For this review, use the dimensioned drawing (mm, ordinates from the lowest corner) and the shaded views. Give positions to 0.01 mm unless a question says otherwise; leave off trailing zeros. Order: outer loops, then holes, each group sorted by start corner. A loop starts at its lowest first (then second) coordinate and runs counter-clockwise, first axis right, second up. Notation, with made-up numbers: M -26.75,35.5 L -1.75,35.5 A8 cw -1.75,47.5 Z; hole C 17.25,35.25 d5. An arc over 180 degrees is marked long. Answer as CSV lines item,"result". Start each with the question number.
1. We need section C-C, the plane y = 1.95. State how many separate pieces and enclosed holes the cut face has, and give its area (3 significant figures).
2. We need section A-A, the plane x = 95. Give the boundary of the cut face in (y, z), and give its area (3 significant figures).
3. We need section B-B, the plane z = 150. Give the boundary of the cut face in (x, y).
4. We need section D-D, the plane z = 49. Give the boundary of the cut face in (x, y).
5. For line 1 along Z through (x, y) = (95, 1.55); line 2 along Z through (x, y) = (108, 2.55) (1 decimal); line 3 along Z through (x, y) = (144, 1.3), list the stretches that pass through material, from the lowest coordinate up.
6. Clearance check with flat-ended pins moving along their axes: P1, Ø2, axis at x = 140, y = 3, coming from the -Z side; P2, Ø1.2, axis at y = 1, z = 113.5, coming from the -X side; P3, Ø1.2, axis at x = 3, y = 1.5, coming from the -Z side; P4, Ø1.2, axis at y = 2.5, z = 7.5, coming from the +X side. State where each tip first meets the part, or that it passes through.
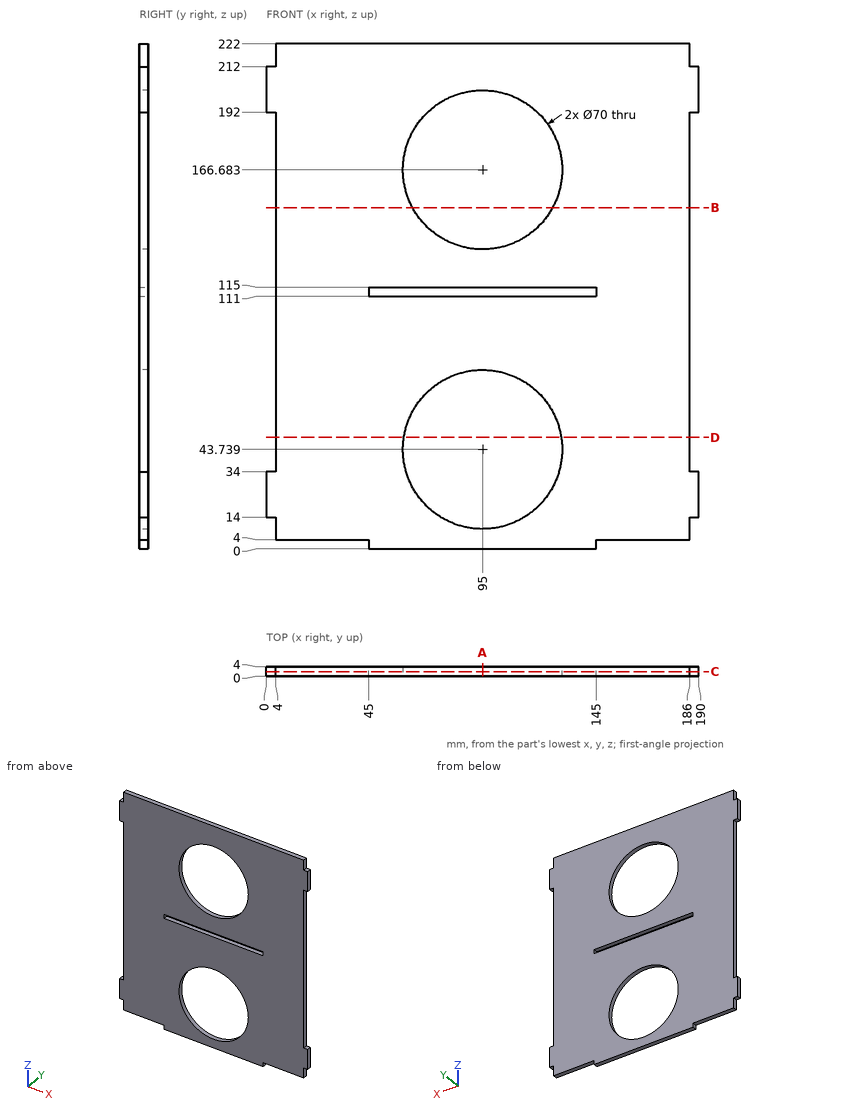
Result set:
1,separate pieces,"1"
1,enclosed holes,"3"
1,area,"32,300 mm2"
2,outline,"M 0,0 L 4,0 L 4,8.74 L 0,8.74 Z; M 0,78.74 L 4,78.74 L 4,111 L 0,111 Z; M 0,115 L 4,115 L 4,131.68 L 0,131.68 Z; M 0,201.68 L 4,201.68 L 4,222 L 0,222 Z"
2,area,"312 mm2"
3,outline,"M 4,0 L 64.23,0 L 64.23,4 L 4,4 Z; M 125.77,0 L 186,0 L 186,4 L 125.77,4 Z"
4,outline,"M 4,0 L 60.4,0 L 60.4,4 L 4,4 Z; M 129.6,0 L 186,0 L 186,4 L 129.6,4 Z"
5,line 1,"0 to 8.74, 78.74 to 111, 115 to 131.68, 201.68 to 222"
5,line 2,"0 to 11.2, 76.2 to 111, 115 to 134.2, 199.2 to 222"
5,line 3,"0 to 111, 115 to 222"
6,P1,"z = 0"
6,P2,"x = 4"
6,P3,"z = 14"
6,P4,"x = 186"
